Check sheet for the modelled part. Datum: model origin and axes. Units: mm. A direction names the side the tool comes from. Round coordinates to 2 decimals unless told otherwise and drop trailing zeros. Write each loop counter-clockwise with the first axis right and the second up, starting at its lowest first coordinate (ties: lowest second). Pieces come first, ordered by that corner, then holes.
Item 1: Cross-section at B-B on z = 1.75. Enter the section's corners in (x, y) (3 decimals), plus the area to 3 significant figures.
Item 2: Cross-section at A-A on y = 0. Enter the section's corners in (x, z) (3 decimals), plus the area to 3 significant figures.
Item 3: Cross-section at C-C on x = 0. Enter the section's corners in (y, z) (3 decimals).
Item 4: Tool access check on faces 1 (the flat face through (-20.038, 0, 2)), 2 (the flat face through (4, -4.038, 2)), 3 (the flat face through (3.038, 4.5, 1.6)). Record the directions out of +Z, -Z, +X, -X, +Y, -Y that give a thin tool (end or side, any length) a straight path to the whole face; none if there is none.
Item 5: Go/stop test with flat-tipped pins: pin 1 Ø4 at (y, z) = (2, 5.5) entering from +X; pin 2 Ø0.5 at (y, z) = (4.5, 1.5) entering from +X; pin 3 Ø2.5 at (x, y) = (-16.875, 0) entering from +Z (3 decimals). Record where each tip stops, or that it passes through.
Item 6: Material ranges on line 1 (Z direction, x = -4.5, y = 0.5) (3 decimals); line 2 (Y direction, x = -13, z = 1.25); line 3 (Y direction, x = -1.5, z = 2.5), recorded low to high.
Item 7: Release check for a two-part mould opening along X. For faces 4 (the cylindrical face through (-0.867, -3.905, 5.196)), 5 (the flat face through (3.038, -4.5, 1.6)), 6 (the cylindrical face through (-11.124, 0.033, 1.565)), 7 (the flat face through (-1, 3, 7.275)) record: +X half, -X half, draft (parallel to the pull), parting line (faces both ways), or undercut.
Item 8: Cross-section at D-D on y = 2.5. Enter the section's corners in (x, z) (1 decimal).
from build123d import *

# Parameters (mm, degrees)
SKETCH1_R           = 2.875
SKETCH1_R_2         = 0.75
BOSS_EXTRUDE1_DEPTH = 3.175
SKETCH2_R           = 4
SKETCH2_R_2         = 2.875
BOSS_EXTRUDE2_DEPTH = 4.1
CUT_EXTRUDE1_DEPTH  = 30.25712561


with BuildPart() as part:
    # Sketch1 → Boss-Extrude1 (new body)
    with BuildSketch(Plane.XY):
        Polygon((-5.038135816, 5.038135816), (-5.038135816, 20.038135816), (5.038135816, 20.038135816), (5.038135816, 5.038135816), (20.038135816, 5.038135816), (20.038135816, -5.038135816), (5.038135816, -5.038135816), (5.038135816, -20.038135816), (-5.038135816, -20.038135816), (-5.038135816, -5.038135816), (-20.038135816, -5.038135816), (-20.038135816, 5.038135816), align=None)
        Circle(SKETCH1_R, mode=Mode.SUBTRACT)
        with Locations((0, 7.125)):
            Circle(SKETCH1_R_2, mode=Mode.SUBTRACT)
        with Locations((0, 10.375)):
            Circle(SKETCH1_R_2, mode=Mode.SUBTRACT)
        with Locations((0, 13.625)):
            Circle(SKETCH1_R_2, mode=Mode.SUBTRACT)
        with Locations((0, 16.875)):
            Circle(SKETCH1_R_2, mode=Mode.SUBTRACT)
        with Locations((7.125, 0)):
            Circle(SKETCH1_R_2, mode=Mode.SUBTRACT)
        with Locations((10.375, 0)):
            Circle(SKETCH1_R_2, mode=Mode.SUBTRACT)
        with Locations((13.625, 0)):
            Circle(SKETCH1_R_2, mode=Mode.SUBTRACT)
        with Locations((16.875, 0)):
            Circle(SKETCH1_R_2, mode=Mode.SUBTRACT)
        with Locations((0, -7.125)):
            Circle(SKETCH1_R_2, mode=Mode.SUBTRACT)
        with Locations((0, -10.375)):
            Circle(SKETCH1_R_2, mode=Mode.SUBTRACT)
        with Locations((0, -13.625)):
            Circle(SKETCH1_R_2, mode=Mode.SUBTRACT)
        with Locations((0, -16.875)):
            Circle(SKETCH1_R_2, mode=Mode.SUBTRACT)
        with Locations((-7.125, 0)):
            Circle(SKETCH1_R_2, mode=Mode.SUBTRACT)
        with Locations((-10.375, 0)):
            Circle(SKETCH1_R_2, mode=Mode.SUBTRACT)
        with Locations((-13.625, 0)):
            Circle(SKETCH1_R_2, mode=Mode.SUBTRACT)
        with Locations((-16.875, 0)):
            Circle(SKETCH1_R_2, mode=Mode.SUBTRACT)
    extrude(amount=BOSS_EXTRUDE1_DEPTH)

    # Sketch2 → Boss-Extrude2 (add)
    with BuildSketch(Plane.XY.offset(3.175)):
        Circle(SKETCH2_R)
        Circle(SKETCH2_R_2, mode=Mode.SUBTRACT)
    extrude(amount=BOSS_EXTRUDE2_DEPTH)

    # Sketch3 → Cut-Extrude1 (cut, through all)
    with BuildSketch(Plane(origin=(0, 0, 0), x_dir=(-1, 0, 0), z_dir=(0, 0, -1))):
        Polygon((-5.038135798, 4.038135816), (-5.038135798, -4.038135816), (-3.038135798, -4.038135816), (-3.038135798, -5.038135816), (5.038135816, -5.038135816), (5.038135816, -21.038135816), (-5.038135816, -21.038135816), (-5.038135816, -5.038135816), (-21.038135816, -5.038135816), (-21.038135816, 5.038135816), (-5.038135816, 5.038135816), (-5.038135816, 21.038135816), (5.038135816, 21.038135816), (5.038135816, 5.038135816), (-3.038135798, 5.038135816), (-3.038135798, 4.038135816), align=None)
    extrude(amount=-CUT_EXTRUDE1_DEPTH, mode=Mode.SUBTRACT)


solid = part.part
Response values:
1. outline: (-20.038, -5.038) - (3.038, -5.038) - (3.038, -4.038) - (5.038, -4.038) - (5.038, 4.038) - (3.038, 4.038) - (3.038, 5.038) - (-20.038, 5.038) - close; hole circle Ø1.5 at (-16.875, 0); hole circle Ø1.5 at (-13.625, 0); hole circle Ø1.5 at (-10.375, 0); hole circle Ø1.5 at (-7.125, 0); hole circle Ø5.75 at (0, 0)
1. area: 216 mm2
2. outline: (-20.038, 0) - (-17.625, 0) - (-17.625, 3.175) - (-20.038, 3.175) - close; (-16.125, 0) - (-14.375, 0) - (-14.375, 3.175) - (-16.125, 3.175) - close; (-12.875, 0) - (-11.125, 0) - (-11.125, 3.175) - (-12.875, 3.175) - close; (-9.625, 0) - (-7.875, 0) - (-7.875, 3.175) - (-9.625, 3.175) - close; (-6.375, 0) - (-2.875, 0) - (-2.875, 7.275) - (-4, 7.275) - (-4, 3.175) - (-6.375, 3.175) - close; (2.875, 0) - (5.038, 0) - (5.038, 3.175) - (4, 3.175) - (4, 7.275) - (2.875, 7.275) - close
2. area: 51.5 mm2
3. outline: (-5.038, 0) - (-2.875, 0) - (-2.875, 7.275) - (-4, 7.275) - (-4, 3.175) - (-5.038, 3.175) - close; (2.875, 0) - (5.038, 0) - (5.038, 3.175) - (4, 3.175) - (4, 7.275) - (2.875, 7.275) - close
4. face 1: +Z, -Z, -X, +Y, -Y
4. face 2: +Z, -Z, +X, -Y
4. face 3: +Z, -Z, +X, +Y
5. pin 1: stops at x = 4
5. pin 2: stops at x = 3.04
5. pin 3: stops at z = 3.175
6. line 1: z = 0 to 3.175
6. line 2: y = -5.04 to -0.41, 0.41 to 5.04
6. line 3: y = -5.04 to -2.45, 2.45 to 5.04
7. face 4: parting line
7. face 5: +X half
7. face 6: undercut
7. face 7: draft
8. outline: (-20, 0) - (-1.4, 0) - (-1.4, 7.3) - (-3.1, 7.3) - (-3.1, 3.2) - (-20, 3.2) - close; (1.4, 0) - (5, 0) - (5, 3.2) - (3.1, 3.2) - (3.1, 7.3) - (1.4, 7.3) - close
